For this review, take the finished solid that the model builds, in its own axes (mm). A direction names the side the tool comes from. Give positions to 0.01 mm unless a question says otherwise; leave off trailing zeros. Order: outer loops, then holes, each group sorted by start corner. A loop starts at its lowest first (then second) coordinate and runs counter-clockwise, first axis right, second up. Notation, with made-up numbers: M 61,-23.75 L 76,-23.75 A14 cw 76,-6.75 Z; hole C -19,60 d6. An arc over 180 degrees is marked long. Answer as CSV lines item,"result". Start each with the question number.
1. Mouldability with a two-part tool opening along X and no side actions: class faces 5 (the flat face through (14.2, 2, 1)), 6 (the flat face through (28, 4.3, 1)) as pulls with the +X half, pulls with the -X half, needs draft (parallel to the pull), parting line crosses it, or undercut.
2. We need section C-C, the plane y = 4.9. Give the boundary of the cut face in (x, z).
3. We need section D-D, the plane x = 30.5. Give the boundary of the cut face in (y, z).
4. For line 1 along X through (y, z) = (3.7, 1.4); line 2 along X through (y, z) = (1.35, 0.2); line 3 along Y through (x, z) = (3.5, 1.4), list the stretches that pass through material, from the lowest coordinate up.
5. We need section A-A, the plane z = 1.3. Give the boundary of the cut face in (x, y), and give its area (3 significant figures).
6. Machinability: for faces 1 (the flat face through (11, 4.3, 1)), 2 (the flat face through (-0.5, 0.5, 2.2)), 3 (the flat face through (24.1, 0.5, 2.2)), 4 (the flat face through (11, 3, 1.9)), which of the approach directions +Z, -Z, +X, -X, +Y, -Y give a long, thin tool a straight path to every point of the face, cutting with its end or side? Answer none if there is none.
7. We need section B-B, the plane x = 24. Give the boundary of the cut face in (y, z), and give its area (3 significant figures).
8. Clearance check with flat-ended pins moving along their axes: P1, Ø0.6, axis at y = 3, z = 1, coming from the +X side; P2, Ø0.6, axis at x = 19, z = 2, coming from the +Y side; P3, Ø1, axis at y = 2.5, z = 1, coming from the -X side. State where each tip first meets the part, or that it passes through.
Autodesk Inventor part; units mm, degrees
ref_plane "YZ Plane" through (0, 0, 0) normal (1, 0, 0) x (0, 1, 0)
ref_plane "XZ Plane" through (0, 0, 0) normal (0, 1, 0) x (-1, 0, 0)
ref_plane "XY Plane" through (0, 0, 0) normal (0, 0, 1) x (1, 0, 0)
sketch "Эскиз1" plane through (0, 0, 0) normal (0, 0, 1) x (1, 0, 0)
  line L0 (0, 0) -> (5.7, 0)
  line L1 (5.7, 0) -> (5.7, 4.3)
  line L2 (5.7, 4.3) -> (0, 4.3)
  line L3 (0, 4.3) -> (0, 0)
  line L4 (8.5, 0) -> (14.2, 0)
  line L5 (14.2, 0) -> (14.2, 4.3)
  line L6 (14.2, 4.3) -> (8.5, 4.3)
  line L7 (8.5, 4.3) -> (8.5, 0)
  line L8 (17, 0) -> (22.7, 0)
  line L9 (22.7, 0) -> (22.7, 4.3)
  line L10 (22.7, 4.3) -> (17, 4.3)
  line L11 (17, 4.3) -> (17, 0)
  line L12 (25.5, 0) -> (31.2, 0)
  line L13 (31.2, 0) -> (31.2, 4.3)
  line L14 (31.2, 4.3) -> (25.5, 4.3)
  line L15 (25.5, 4.3) -> (25.5, 0)
  dimension "d0" = 4.3
  dimension "d1" = 5.7
  dimension "d4" = 8.5
extrude "Выдавливание1" add sketch "Эскиз1" along normal blind 2.4
sketch "Эскиз2" plane through (0, 0, 2.4) normal (0, 0, 1) x (1, 0, 0)
  line L0 (-1, 4.3) -> (32.2, 4.3)
  line L1 (32.2, 4.3) -> (32.2, 5.2)
  line L2 (32.2, 5.2) -> (-1, 5.2)
  line L3 (-1, 5.2) -> (-1, 4.3)
  line L4 (-1, 0) -> (32.2, 0)
  line L5 (32.2, 0) -> (32.2, 0.9)
  line L6 (32.2, 0.9) -> (-1, 0.9)
  line L7 (-1, 0.9) -> (-1, 0)
  line L8 (5.7, 4.3) -> (0, 4.3)
  line L9 (0, 4.3) -> (5.7, 4.3)
  line L10 (5.7, 4.3) -> (5.7, 4.3)
  line L11 (5.7, 4.3) -> (0, 4.3)
  line L12 (0, 4.3) -> (0, 4.3)
  line L13 (14.2, 4.3) -> (8.5, 4.3)
  line L14 (8.5, 4.3) -> (14.2, 4.3)
  line L15 (14.2, 4.3) -> (14.2, 4.3)
  line L16 (14.2, 4.3) -> (8.5, 4.3)
  line L17 (8.5, 4.3) -> (8.5, 4.3)
  line L18 (17, 4.3) -> (22.7, 4.3)
  line L19 (22.7, 4.3) -> (22.7, 4.3)
  line L20 (22.7, 4.3) -> (17, 4.3)
  line L21 (17, 4.3) -> (17, 4.3)
  line L22 (31.2, 4.3) -> (25.5, 4.3)
  line L23 (25.5, 4.3) -> (31.2, 4.3)
  line L24 (31.2, 4.3) -> (31.2, 4.3)
  line L25 (31.2, 4.3) -> (25.5, 4.3)
  line L26 (25.5, 4.3) -> (25.5, 4.3)
  line L27 (0, 4.3) -> (0, 0)
  line L28 (31.2, 0) -> (31.2, 4.3)
  point P0 (31.2, 0.9)
  point P1 (0, 0.9)
  point P2 (25.5, 4.8)
  point P3 (17, 4.8)
  point P4 (0, 4.8)
  point P5 (8.5, 4.8)
  dimension "d11" = 0.9
  dimension "d12" = 0
  dimension "d13" = 0.9
  dimension "d14" = 1
  dimension "d15" = 1
extrude "Выдавливание2" add sketch "Эскиз2" against normal blind 0.2 contours L3 L2 L1 L0 | L27 L4 L7 L6 | L6 L28 L4 L27 | L6 L5 L4 L28
sketch "Эскиз3" plane through (0, 0, 2.4) normal (0, 0, 1) x (1, 0, 0)
  line L0 (32.2, 5.2) -> (-1, 5.2)
  line L1 (1.15, 1) -> (4.55, 1)
  line L2 (4.55, 1) -> (4.55, 5.2)
  line L3 (4.55, 5.2) -> (1.15, 5.2)
  line L4 (1.15, 5.2) -> (1.15, 1)
  line L5 (0, 4.3) -> (5.7, 4.3)
  line L6 (9.65, 1) -> (13.05, 1)
  line L7 (13.05, 1) -> (13.05, 5.2)
  line L8 (13.05, 5.2) -> (9.65, 5.2)
  line L9 (9.65, 5.2) -> (9.65, 1)
  line L10 (18.15, 1) -> (21.55, 1)
  line L11 (21.55, 1) -> (21.55, 5.2)
  line L12 (21.55, 5.2) -> (18.15, 5.2)
  line L13 (18.15, 5.2) -> (18.15, 1)
  line L14 (26.65, 1) -> (30.05, 1)
  line L15 (30.05, 1) -> (30.05, 5.2)
  line L16 (30.05, 5.2) -> (26.65, 5.2)
  line L17 (26.65, 5.2) -> (26.65, 1)
  point P0 (0, 0)
  point P1 (2.85, 4.3)
  point P2 (2.85, 1)
  point P3 (11.35, 1)
  point P4 (11.35, 4.3)
  point P5 (19.85, 1)
  point P6 (19.85, 4.3)
  point P7 (28.35, 1)
  point P8 (28.35, 4.3)
  point P9 (13.05, 5.2)
  point P10 (21.55, 5.2)
  point P11 (30.05, 5.2)
  dimension "d18" = 3.4
  dimension "d19" = 4.2
  dimension "d22" = 8.5
extrude "Выдавливание3" cut sketch "Эскиз3" against normal blind 0.5
chamfer "Фаска1" distance 0.4 angle 45 16 edges at (2.85, 4.3, 0) (0, 2.15, 0) (2.85, 0, 0) (5.7, 2.15, 0) (8.5, 2.15, 0) (11.35, 4.3, 0) (14.2, 2.15, 0) (11.35, 0, 0) (19.85, 0, 0) (17, 2.15, 0) (19.85, 4.3, 0) (22.7, 2.15, 0) (25.5, 2.15, 0) (28.35, 4.3, 0) (31.2, 2.15, 0) (28.35, 0, 0)
properties part number "buttons"
Result set:
1,face 5,"undercut"
1,face 6,"needs draft"
2,outline,"M -1,2.2 L 1.15,2.2 L 1.15,2.4 L -1,2.4 Z; M 4.55,2.2 L 9.65,2.2 L 9.65,2.4 L 4.55,2.4 Z; M 13.05,2.2 L 18.15,2.2 L 18.15,2.4 L 13.05,2.4 Z; M 21.55,2.2 L 26.65,2.2 L 26.65,2.4 L 21.55,2.4 Z; M 30.05,2.2 L 32.2,2.2 L 32.2,2.4 L 30.05,2.4 Z"
3,outline,"M 0,0.4 L 0.4,0 L 3.9,0 L 4.3,0.4 L 4.3,2.2 L 5.2,2.2 L 5.2,2.4 L 0,2.4 Z"
4,line 1,"0 to 5.7, 8.5 to 14.2, 17 to 22.7, 25.5 to 31.2"
4,line 2,"0.2 to 5.5, 8.7 to 14, 17.2 to 22.5, 25.7 to 31"
4,line 3,"0 to 4.3"
5,outline,"M 0,0 L 5.7,0 L 5.7,4.3 L 0,4.3 Z; M 8.5,0 L 14.2,0 L 14.2,4.3 L 8.5,4.3 Z; M 17,0 L 22.7,0 L 22.7,4.3 L 17,4.3 Z; M 25.5,0 L 31.2,0 L 31.2,4.3 L 25.5,4.3 Z"
5,area,"98.0 mm2"
6,face 1,"-Z, +X, -X, +Y"
6,face 2,"-Z, -X, +Y, -Y"
6,face 3,"-Z, +Y, -Y"
6,face 4,"+Z, +Y"
7,outline,"M 0,2.2 L 0.9,2.2 L 0.9,2.4 L 0,2.4 Z; M 4.3,2.2 L 5.2,2.2 L 5.2,2.4 L 4.3,2.4 Z"
7,area,"0.360 mm2"
8,P1,"x = 31.2"
8,P2,"y = 4.3"
8,P3,"x = 0"
